Check sheet for the modelled part. Datum: model origin and axes. Units: mm. Round coordinates to 2 decimals unless told otherwise and drop trailing zeros. Write each loop counter-clockwise with the first axis right and the second up, starting at its lowest first coordinate (ties: lowest second). Pieces come first, ordered by that corner, then holes.
Item 1: Section check A-A, the plane y = 3. Record the cut outline in (x, z).
Item 2: Section check C-C, the plane x = 61.5. Record the cut outline in (y, z).
Item 3: Section check B-B, the plane z = 23. Record the cut outline in (x, y).
Item 4: Section check D-D, the plane z = 33.5. Record the cut outline in (x, y).
Item 5: Material ranges on line 1 along Y through (x, z) = (-71.5, 39.5) (3 decimals); line 2 along X through (y, z) = (-10, 25); line 3 along X through (y, z) = (-2, 6), recorded low to high.
Item 6: Depth check by flat-ended pin: pin 1 (12 mm diameter, centred on x = -24, y = 25, fed in from +Z); pin 2 (5 mm diameter, centred on y = -5.5, z = 32, fed in from +X); pin 3 (2 mm diameter, centred on y = 16, z = 53.5, fed in from +X). Enter the tip coordinate at first touch or a pass-through.
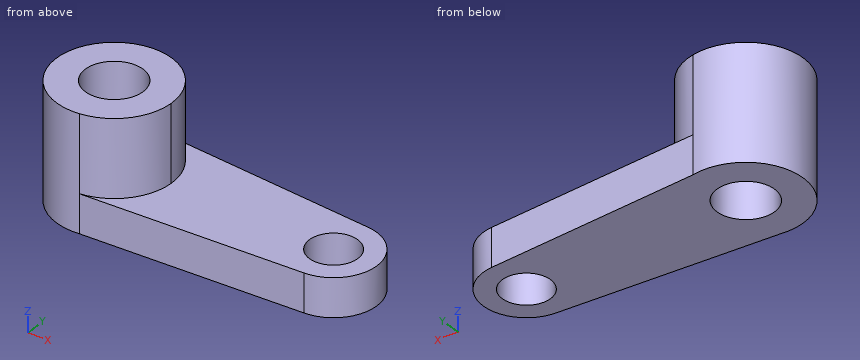
from build123d import *

# Parameters (mm, degrees)
F0_R     = 16.087734
F1_DEPTH = 25.4
F0_R_2   = 19.193831
F2_DEPTH = 76.2


with BuildPart() as f1:
    # F0 (on Top) → F1 (new body)
    with BuildSketch(Plane.XY):
        with BuildLine():
            ThreePointArc((-65.353721, 37.574831), (-42.954198, 24.427618), (-34.129272, 0))
            ThreePointArc((-34.129272, 0), (-43.542934, -25.119206), (-67.146784, -37.864785))
            Line((-67.146784, -37.864785), (76.868893, -28.595699))
            ThreePointArc((76.868893, -28.595699), (103.683287, 0.017515), (76.833934, 28.597927))
            Line((76.833934, 28.597927), (-65.353721, 37.574831))
        make_face()
        with Locations((75.028427, 0)):
            Circle(F0_R, mode=Mode.SUBTRACT)
    extrude(amount=F1_DEPTH)

    # F0 (on Top) → F2 (join)
    with BuildSketch(Plane.XY):
        with BuildLine():
            ThreePointArc((-67.146784, -37.864785), (-43.542934, -25.119206), (-34.129272, 0))
            ThreePointArc((-34.129272, 0), (-42.954198, 24.427618), (-65.353721, 37.574831))
            ThreePointArc((-65.353721, 37.574831), (-110.559674, 0.908178), (-67.146784, -37.864785))
        make_face()
        with Locations((-72.349869, 0)):
            Circle(F0_R_2, mode=Mode.SUBTRACT)
    extrude(amount=F2_DEPTH)


solid = f1.part
Values found:
1. outline: (-110.45, 0) - (-91.31, 0) - (-91.31, 76.2) - (-110.45, 76.2) - close; (-53.39, 0) - (59.22, 0) - (59.22, 25.4) - (-34.25, 25.4) - (-34.25, 76.2) - (-53.39, 76.2) - close; (90.83, 0) - (103.53, 0) - (103.53, 25.4) - (90.83, 25.4) - close
2. outline: (-29.58, 0) - (-8.71, 0) - (-8.71, 25.4) - (-29.58, 25.4) - close; (8.71, 0) - (29.57, 0) - (29.57, 25.4) - (8.71, 25.4) - close
3. outline: (-67.15, -37.86) - (76.87, -28.6) arc R28.65 ccw to (76.83, 28.6) - (-65.35, 37.57) arc R38.22 ccw (long way) to start; hole circle Ø38.39 at (-72.35, 0); hole circle Ø32.18 at (75.03, 0)
4. outline: (-67.15, -37.86) arc R38.22 ccw to (-34.13, 0) arc R38.22 ccw to (-65.35, 37.57) arc R38.22 ccw (long way) to start; hole circle Ø38.39 at (-72.35, 0)
5. line 1: y = -38.211 to -19.175, 19.175 to 38.211
5. line 2: x = -109.24 to -88.73, -55.97 to 62.43, 87.63 to 101.88
5. line 3: x = -110.52 to -91.44, -53.26 to 59.07, 90.99 to 103.61
6. pin 1: stops at z = 25.4
6. pin 2: stops at x = -34.25
6. pin 3: stops at x = -37.2
